Design review of the part built by this model. Coordinates are the model's own, in mm. A direction names the side the tool comes from. Give positions to 0.01 mm unless a question says otherwise; leave off trailing zeros. Write each loop counter-clockwise with the first axis right and the second up, starting at its lowest first coordinate (ties: lowest second). Pieces come first, ordered by that corner, then holes.
```python
from build123d import *

# Parameters (mm, degrees)
SKETCH1_R          = 3
SKETCH1_R_2        = 2
SKETCH1_W          = 15
SKETCH1_H          = 3.175
BASE_FLANGE1_DEPTH = 3.175


# Sheet-metal steps are written as plain solids
with BuildPart() as part:
    # Sketch1 → Base-Flange1 (new body)
    with BuildSketch(Plane.XY):
        Polygon((-1.53, -68.5), (25.47, -95.5), (185, -95.5), (185, -143.5), (185, -148.5), (185, -152.205), (41.281460478, -152.205), (41.281460478, -172.205), (-8.718539522, -172.205), (-8.718539522, -152.205), (-15, -152.205), (-15, -150.03), (-15, -83.5), (-55, -83.5), (-55, -68.5), align=None)
        with Locations((1.281460478, -162.205)):
            Circle(SKETCH1_R, mode=Mode.SUBTRACT)
        with Locations((31.281460478, -162.205)):
            Circle(SKETCH1_R, mode=Mode.SUBTRACT)
        with Locations((-42.5, -76)):
            Circle(SKETCH1_R_2, mode=Mode.SUBTRACT)
        with Locations((-12.5, -76)):
            Circle(SKETCH1_R_2, mode=Mode.SUBTRACT)
        with Locations((-11, -141.03)):
            Circle(SKETCH1_R_2, mode=Mode.SUBTRACT)
        with Locations((160, -146.6175)):
            Rectangle(SKETCH1_W, SKETCH1_H, mode=Mode.SUBTRACT)
        with Locations((40, -146.6175)):
            Rectangle(SKETCH1_W, SKETCH1_H, mode=Mode.SUBTRACT)
        with Locations((0, -146.6175)):
            Rectangle(SKETCH1_W, SKETCH1_H, mode=Mode.SUBTRACT)
        Polygon((0, -84.172135624), (11.327864376, -95.5), (0, -95.5), align=None, mode=Mode.SUBTRACT)
        with Locations((80, -146.6175)):
            Rectangle(SKETCH1_W, SKETCH1_H, mode=Mode.SUBTRACT)
        with Locations((120, -146.6175)):
            Rectangle(SKETCH1_W, SKETCH1_H, mode=Mode.SUBTRACT)
        with BuildLine():
            Line((104.058089569, -112.488390285), (159.709824243, -112.488390285))
            ThreePointArc((159.709824243, -112.488390285), (167.979359115, -120.757925156), (159.709824243, -129.027460028))
            Line((159.709824243, -129.027460028), (104.058089569, -129.027460028))
            ThreePointArc((104.058089569, -129.027460028), (95.788554697, -120.757925156), (104.058089569, -112.488390285))
        make_face(mode=Mode.SUBTRACT)
        with BuildLine():
            Line((15.775217294, -112.93539217), (71.426951968, -112.93539217))
            ThreePointArc((71.426951968, -112.93539217), (79.69648684, -121.204927041), (71.426951968, -129.474461913))
            Line((71.426951968, -129.474461913), (15.775217294, -129.474461913))
            ThreePointArc((15.775217294, -129.474461913), (7.505682422, -121.204927041), (15.775217294, -112.93539217))
        make_face(mode=Mode.SUBTRACT)
        with BuildLine():
            Line((181, -102.5), (179, -102.5))
            ThreePointArc((179, -102.5), (177, -100.5), (179, -98.5))
            Line((179, -98.5), (181, -98.5))
            ThreePointArc((181, -98.5), (183, -100.5), (181, -102.5))
        make_face(mode=Mode.SUBTRACT)
        with BuildLine():
            Line((171, -102.5), (169, -102.5))
            ThreePointArc((169, -102.5), (167, -100.5), (169, -98.5))
            Line((169, -98.5), (171, -98.5))
            ThreePointArc((171, -98.5), (173, -100.5), (171, -102.5))
        make_face(mode=Mode.SUBTRACT)
        with BuildLine():
            Line((171, -128.5), (169, -128.5))
            ThreePointArc((169, -128.5), (167, -130.5), (169, -132.5))
            Line((169, -132.5), (171, -132.5))
            ThreePointArc((171, -132.5), (173, -130.5), (171, -128.5))
        make_face(mode=Mode.SUBTRACT)
        with BuildLine():
            Line((181, -128.5), (179, -128.5))
            ThreePointArc((179, -128.5), (177, -130.5), (179, -132.5))
            Line((179, -132.5), (181, -132.5))
            ThreePointArc((181, -132.5), (183, -130.5), (181, -128.5))
        make_face(mode=Mode.SUBTRACT)
    extrude(amount=-BASE_FLANGE1_DEPTH)


solid = part.part
```
(1) Clearance check with flat-ended pins moving along their axes: P1, Ø1, axis at x = 6.5, z = -1.5, coming from the +Y side; P2, Ø1.6, axis at x = 170, z = -1, coming from the +Y side; P3, Ø1, axis at y = -88.5, z = -1.5, coming from the +X side; P4, Ø5, axis at x = 1.28, y = -162.21, coming from the -Z side. State where each tip first meets the part, or that it passes through.
Resolved:
P1: stops at y = -76.03
P2: stops at y = -95.5
P3: stops at x = 18.97
P4: passes through
(2) Consider section A-A, the plane x = -30. Give the boundary of the cut face in (y, z) (3 decimals).
Resolved:
outline: (-83.5, -3.175) - (-68.5, -3.175) - (-68.5, 0) - (-83.5, 0) - close
(3) Mouldability with a two-part tool opening along X and no side actions: class faces 3 (the face through (67, -108, -3.175)), 4 (the face through (-11.26, -139.047, -1.565)), 5 (the face through (11.78, -81.81, -1.57)) as pulls with the +X half, pulls with the -X half, needs draft (parallel to the pull), parting line crosses it, or undercut.
Resolved:
face 3: needs draft
face 4: undercut
face 5: pulls with the +X half
(4) Consider section B-B, the plane z = -1.15. Give the number of separate pieces and of enclosed holes in the cut face, then the cut area to 3 significant figures.
Resolved:
separate pieces: 1
enclosed holes: 17
area: 10,900 mm2
(5) Tool access review of faces 1 (the face through (67, -108, 0)), 2 (the face through (79.694, -121.023, -1.565)): name each direction out of +Z, -Z, +X, -X, +Y, -Y from which nothing blocks a thin tool from reaching the whole face with its end or side.
Resolved:
face 1: +Z, +X, -X, +Y, -Y
face 2: +Z, -Z
(6) To check wall thickness, follow L1, parallel to Y at x = 119, z = -0.7 (3 decimals); L2, parallel to Y at x = -42.5, z = -1.1; L3, parallel to Y at x = -12.5, z = -1.4 (3 decimals). State the ranges of each line that lie inside material, in increasing order.
Resolved:
L1: y = -152.205 to -148.205, -145.03 to -129.027, -112.488 to -95.5
L2: y = -83.5 to -78, -74 to -68.5
L3: y = -152.205 to -142.353, -139.707 to -78, -74 to -68.5
